Autodesk Inventor part; units mm, degrees
ref_plane "YZ Plane" through (0, 0, 0) normal (1, 0, 0) x (0, 1, 0)
ref_plane "XZ Plane" through (0, 0, 0) normal (0, 1, 0) x (-1, 0, 0)
ref_plane "XY Plane" through (0, 0, 0) normal (0, 0, 1) x (1, 0, 0)
sketch "Sketch1" plane through (0, 0, 0) normal (0, 1, 0) x (-1, 0, 0)
  line L0 (0, 0) -> (12.7, 0)
  line L1 (12.7, 0) -> (12.7, -76.2)
  line L2 (12.7, -76.2) -> (0, -76.2)
  line L3 (0, -76.2) -> (0, 0)
  dimension "d0" = 12.7
  dimension "d1" = 76.2
extrude "Extrusion1" add sketch "Sketch1" along normal blind 76.2
sketch "Sketch2" plane through (0, 0, 0) normal (0, -1, 0) x (1, 0, 0)
  circle A0 centre (-6.35, -25.4) radius 1.27
  circle A1 centre (-6.35, -50.8) radius 1.27
  line L0 (0, 0) -> (-12.7, 0)
  line L1 (-12.7, -76.2) -> (0, -76.2)
  dimension "d4" = 2.54
  dimension "d5" = 2.54
  dimension "d6" = 25.4
  dimension "d8" = 25.4
  dimension "d9" = 6.35
extrude "Extrusion2" cut sketch "Sketch2" against normal blind 6.35
sketch "Sketch3" plane through (0, 0, 0) normal (1, 0, 0) x (0, 0, -1)
  circle A0 centre (38.1, 41.275) radius 6.35
  circle A1 centre (25.4, 41.275) radius 2.54
  line L0 (0, 0) -> (0, 76.2)
  circle A2 centre (50.8, 41.275) radius 2.54
  line L1 (76.2, 0) -> (0, 0)
  dimension "d12" = 12.7
  dimension "d13" = 5.08
  dimension "d15" = 38.1
  dimension "d16" = 25.4
  dimension "d19" = 360
  dimension "d21" = 41.275
extrude "Extrusion3" cut sketch "Sketch3" against normal up to next
thread "Thread1"
thread "Thread2"
chamfer "Chamfer1" distance 0.254 angle 45 18 edges at (0, 41.275, -31.75) (0, 41.275, -22.86) (0, 41.275, -48.26) (-12.7, 41.275, -48.26) (-12.7, 41.275, -31.75) (-12.7, 41.275, -22.86) (0, 76.2, -38.1) (-6.35, 76.2, 0) (-12.7, 76.2, -38.1) (0, 38.1, 0) (-12.7, 38.1, 0) (0, 38.1, -76.2) (0, 0, -38.1) (-6.35, 0, 0) (-12.7, 38.1, -76.2) (-12.7, 0, -38.1) (-6.35, 76.2, -76.2) (-6.35, 0, -76.2)
properties part number "Fixture-Center"
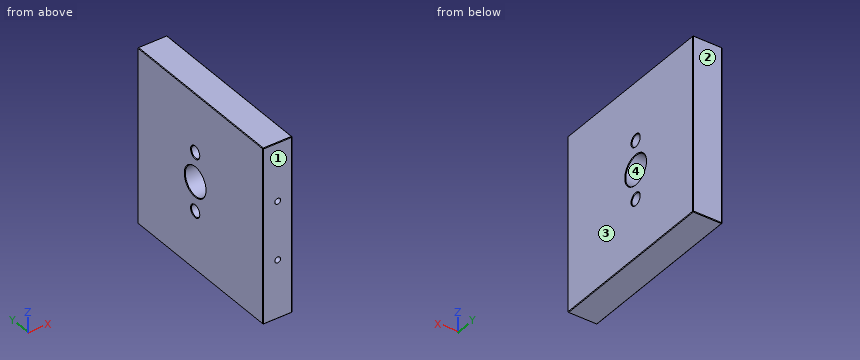
CAD build for the part. Positions are in the model's coordinates, mm. Face numbers are marked on the shaded views. Give positions to 0.01 mm unless a question says otherwise; leave off trailing zeros. Order: outer loops, then holes, each group sorted by start corner. A loop starts at its lowest first (then second) coordinate and runs counter-clockwise, first axis right, second up. Notation, with made-up numbers: (-0.5, -28.5) -> (6.5, -28.5) arc R24 cw to (6.5, 10.5) -> close; hole circle Ø3 at (83.25, -2.75). An arc over 180 degrees is marked (long way). Return JSON: item names as keys, results as strings.
Q1. Flat gauge pin, fed straight in: pin 1 (0.8 mm diameter, centred on x = -6.5, z = -26, fed in from -Y). Where does the tip first touch, or does it go through?
Working result:
{"pin 1": "y = 6.35"}
Q2. Saw through at D-D (x = -6.35). Write the cut outline in (y, z) (3 decimals), then the cut area to 3 significant figures.
Working result:
{"outline": "(0, -75.946) -> (0.254, -76.2) -> (75.946, -76.2) -> (76.2, -75.946) -> (76.2, -0.254) -> (75.946, 0) -> (0.254, 0) -> (0, -0.254) -> (0, -24.13) -> (6.35, -24.13) -> (6.35, -26.67) -> (0, -26.67) -> (0, -49.53) -> (6.35, -49.53) -> (6.35, -52.07) -> (0, -52.07) -> close; hole circle Ø12.7 at (41.275, -38.1); hole circle Ø5.08 at (41.275, -50.8); hole circle Ø5.08 at (41.275, -25.4)", "area": "5,610 mm²"}
Q3. Saw through at B-B (x = -1.5). Write the cut outline in (y, z) (3 decimals).
Working result:
{"outline": "(0, -75.946) -> (0.254, -76.2) -> (75.946, -76.2) -> (76.2, -75.946) -> (76.2, -0.254) -> (75.946, 0) -> (0.254, 0) -> (0, -0.254) -> close; hole circle Ø12.7 at (41.275, -38.1); hole circle Ø5.08 at (41.275, -50.8); hole circle Ø5.08 at (41.275, -25.4)"}
Q4. Saw through at C-C (z = -38.1). Write the cut outline in (x, y) (3 decimals), then the cut area to 3 significant figures.
Working result:
{"outline": "(-12.7, 0.254) -> (-12.446, 0) -> (-0.254, 0) -> (0, 0.254) -> (0, 34.671) -> (-0.254, 34.925) -> (-12.446, 34.925) -> (-12.7, 34.671) -> close; (-12.7, 47.879) -> (-12.446, 47.625) -> (-0.254, 47.625) -> (0, 47.879) -> (0, 75.946) -> (-0.254, 76.2) -> (-12.446, 76.2) -> (-12.7, 75.946) -> close", "area": "806 mm²"}
Q5. Saw through at A-A (z = -25.4). Write the cut outline in (x, y) (3 decimals).
Working result:
{"outline": "(-12.7, 0.254) -> (-12.446, 0) -> (-7.62, 0) -> (-7.62, 6.35) -> (-5.08, 6.35) -> (-5.08, 0) -> (-0.254, 0) -> (0, 0.254) -> (0, 38.481) -> (-0.254, 38.735) -> (-12.446, 38.735) -> (-12.7, 38.481) -> close; (-12.7, 44.069) -> (-12.446, 43.815) -> (-0.254, 43.815) -> (0, 44.069) -> (0, 75.946) -> (-0.254, 76.2) -> (-12.446, 76.2) -> (-12.7, 75.946) -> close"}
Q6. Mould opens along Y. For the marked faces 1, 2, 3 and 4 say: pulls with the +Y half, pulls with the -Y half, needs draft (parallel to the pull), parting line crosses it, or undercut.
Working result:
{"face 1": "pulls with the -Y half", "face 2": "pulls with the +Y half", "face 3": "needs draft", "face 4": "undercut"}
Q7. Drill centre lines: line 1 (Z direction, x = -6.35, y = 2.75); line 2 (Y direction, x = -5, z = -38.1) (3 decimals); line 3 (Z direction, x = -4, y = 41). Where is each one in solid material? Low to high.
Working result:
{"line 1": "-76.2 to -52.07, -49.53 to -26.67, -24.13 to 0", "line 2": "0 to 34.925, 47.625 to 76.2", "line 3": "-76.2 to -53.33, -48.27 to -44.44, -31.76 to -27.93, -22.87 to 0"}
